Study the drawing (mm; zero at the part's minimum x, y, z) and answer. Give positions to 0.01 mm unless a question says otherwise; leave off trailing zeros. Order: outer loops, then holes, each group sorted by start corner. A loop starts at its lowest first (then second) coordinate and runs counter-clockwise, first axis right, second up. Notation, with made-up numbers: (9, 57) - (18, 57) arc R21 ccw to (18, 90) - close; hole circle Ø3 at (-28, 47). An arc over 180 degrees is marked (long way). Use CSV: the item, a comma, the result in double quotes.
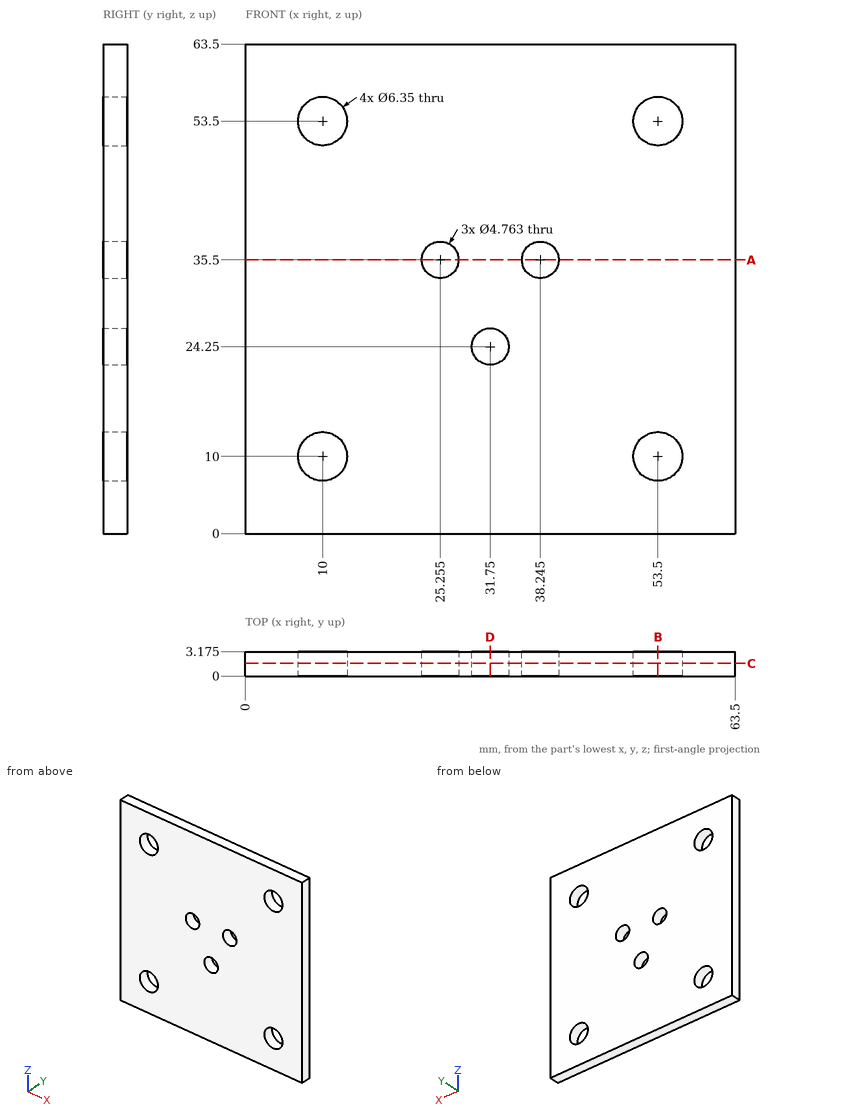
Item 1: This flat-tipped pin is pushed along its axis until it touches: pin 1 (5 mm diameter, centred on x = 23, z = 17, fed in from -Y). Where does it stop, or does it pass through?
Taken from the geometry:
pin 1,"y = 0"
Item 2: The part is cut by section B-B (x = 53.5). Give the vertices of the cut face in (y, z) (1 decimal), and give its area (3 significant figures).
Taken from the geometry:
outline,"(0, 0) - (3.2, 0) - (3.2, 6.8) - (0, 6.8) - close; (0, 13.2) - (3.2, 13.2) - (3.2, 50.3) - (0, 50.3) - close; (0, 56.7) - (3.2, 56.7) - (3.2, 63.5) - (0, 63.5) - close"
area,"161 mm^2"
Item 3: The part is cut by section A-A (z = 35.5). Give the vertices of the cut face in (x, y) (1 decimal), and give its area (3 significant figures).
Taken from the geometry:
outline,"(0, 0) - (22.9, 0) - (22.9, 3.2) - (0, 3.2) - close; (27.6, 0) - (35.9, 0) - (35.9, 3.2) - (27.6, 3.2) - close; (40.6, 0) - (63.5, 0) - (63.5, 3.2) - (40.6, 3.2) - close"
area,"171 mm^2"
Item 4: The part is cut by section C-C (y = 1.65). Count the separate pieces of the cut face and the enclosed holes in it, and give its area (3 significant figures).
Taken from the geometry:
separate pieces,"1"
enclosed holes,"7"
area,"3,850 mm^2"
Item 5: Find the intervals of material crossed by line 1 along X through (y, z) = (1.15, 35.5); line 2 along Z through (x, y) = (53.5, 1.2) (1 decimal); line 3 along Z through (x, y) = (51, 0.4) (1 decimal), in increasing order.
Taken from the geometry:
line 1,"0 to 22.87, 27.64 to 35.86, 40.63 to 63.5"
line 2,"0 to 6.8, 13.2 to 50.3, 56.7 to 63.5"
line 3,"0 to 8, 12 to 51.5, 55.5 to 63.5"
Item 6: The part is cut by section D-D (x = 31.75). Give the vertices of the cut face in (y, z) (1 decimal).
Taken from the geometry:
outline,"(0, 0) - (3.2, 0) - (3.2, 21.9) - (0, 21.9) - close; (0, 26.6) - (3.2, 26.6) - (3.2, 63.5) - (0, 63.5) - close"
